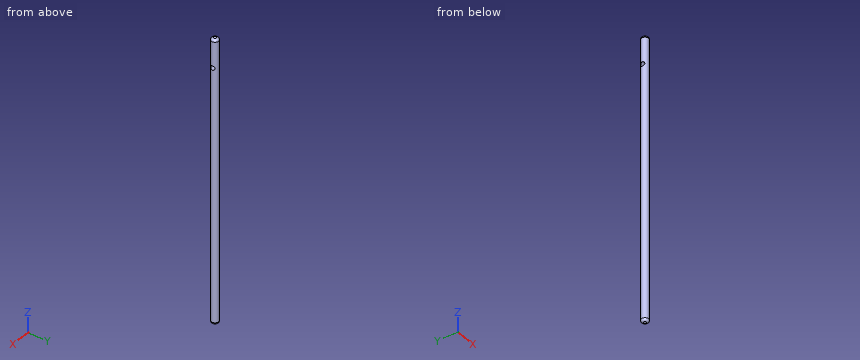
from build123d import *

# Parameters (mm, degrees)
BOSS_EXTRUDE1_DEPTH      = 500
BOSS_EXTRUDE1_DEPTH_BACK = 500
SKETCH1_R                = 12.7
FILLET1_R                = 8
CUT_EXTRUDE1_DEPTH       = 15
CUT_EXTRUDE1_DEPTH_BACK  = 19
SKETCH3_R                = 7.5


with BuildPart() as part:
    # Sketch1 → Boss-Extrude1 (new, two sides: drawn at the far end of the back side and taken through both)
    with BuildSketch(Plane.XY.offset(-BOSS_EXTRUDE1_DEPTH_BACK)):
        Circle(SKETCH1_R)
    extrude(amount=BOSS_EXTRUDE1_DEPTH + BOSS_EXTRUDE1_DEPTH_BACK)

    # Fillet1
    fillet1_edges = [part.edges().sort_by_distance(p)[0] for p in [
        (-12.7, 0, 500),
        (-12.7, 0, -500),
    ]]
    fillet(fillet1_edges, radius=FILLET1_R)

    # Sketch3 → Cut-Extrude1 (cut, two sides: drawn at the far end of the back side and taken through both)
    with BuildSketch(Plane(origin=(0, 0, 0), x_dir=(0, 0, -1), z_dir=(1, 0, 0)).offset(-CUT_EXTRUDE1_DEPTH_BACK)):
        with Locations(Location((-400, 0.2, 0), (0, 0, 180))):
            Circle(SKETCH3_R)
    extrude(amount=CUT_EXTRUDE1_DEPTH + CUT_EXTRUDE1_DEPTH_BACK, mode=Mode.SUBTRACT)


solid = part.part
Design review of the part built by this model. Coordinates are the model's own, in mm. Give positions to 0.01 mm unless a question says otherwise; leave off trailing zeros. Loops run counter-clockwise (first coordinate to the right, second up) from the corner with the lowest first, then second, coordinate; pieces in that order, holes last. Notation, with made-up numbers: M 60,51.5 L 96,51.5 A23 ccw 96,79.5 Z; hole C 60.25,-26 d5. An arc over 180 degrees is marked long. Answer as a JSON object with one key per item and string values.
Item 1: Wall thickness on line 1 along Y through (x, z) = (0.5, 400); line 2 along Z through (x, y) = (-5.5, 0.25); line 3 along X through (y, z) = (-0.75, 132): over which ranges is each line inside the solid? List them lowest first.
Output values:
{"line 1": "y = -12.69 to -7.3, 7.7 to 12.69", "line 2": "z = -499.96 to 392.5, 407.5 to 499.96", "line 3": "x = -12.68 to 12.68"}
Item 2: We need section A-A (z = -68.5). State the section outline as (x, y) points.
Output values:
{"outline": "C 0,0 d25.4"}
Item 3: For P1, Ø2, axis at y = -5, z = -302.5, coming from the -X side; P2, Ø4, axis at x = -3, z = 133.5, coming from the +Y side; P3, Ø9, axis at y = 0.2, z = 400, coming from the -X side; P4, Ø1.5, axis at x = 7.5, y = 4, coming from the +Z side, all flat-tipped, find the tip position at first contact; note any pin that passes through.
Output values:
{"P1": "stops at x = -12.05", "P2": "stops at y = 12.66", "P3": "passes through", "P4": "stops at z = 499.4"}
